For this review, take the finished solid that the model builds, in its own axes (mm). A direction names the side the tool comes from. Give positions to 0.01 mm unless a question says otherwise; leave off trailing zeros. Order: outer loops, then holes, each group sorted by start corner. A loop starts at its lowest first (then second) coordinate and runs counter-clockwise, first axis right, second up. Notation, with made-up numbers: (87.25, 33.25) - (144.25, 33.25) arc R12 ccw to (144.25, 54.25) - close; hole circle Ø5 at (-14.75, 64). An arc over 180 degrees is marked (long way). One line per item, written item: value.
```python
from build123d import *

# Parameters (mm, degrees)
ESBO_O1_R             = 1.25
CORTE_EXTRUS_O1_DEPTH = 10


with BuildPart() as part:
    # Sketch1 → Revolve1 (revolve)
    with BuildSketch(Plane(origin=(0, 0, 0), x_dir=(1, 0, 0), z_dir=(0, 1, 0))):
        Polygon((0, 0), (7, 0), (41.5, 0), (53.5, 0), (53.5, 3), (41.5, 3), (41.5, 3.05), (7, 3.05), (7, 3), (0, 3), align=None)
    revolve(axis=Axis((0, 0, 0), (-1, 0, 0)))

    # Esboço1 → Corte-extrusão1 (cut)
    with BuildSketch(Plane(origin=(53.5, 0, 0), x_dir=(0, 0, -1), z_dir=(1, 0, 0))):
        Circle(ESBO_O1_R)
    extrude(amount=-CORTE_EXTRUS_O1_DEPTH, mode=Mode.SUBTRACT)


solid = part.part
```
(1) For P1, Ø3, axis at x = 44, z = -1.5, coming from the -Y side; P2, Ø1.2, axis at y = -0.5, z = 0, coming from the +X side, all flat-tipped, find the tip position at first contact; note any pin that passes through.
Answers below:
P1: stops at y = -3
P2: stops at x = 43.5
(2) Take a section at A-A (z = 0). Write out the cut boundary in (x, y).
Answers below:
outline: (0, -3) - (7, -3) - (7, -3.05) - (41.5, -3.05) - (41.5, -3) - (53.5, -3) - (53.5, -1.25) - (43.5, -1.25) - (43.5, 1.25) - (53.5, 1.25) - (53.5, 3) - (41.5, 3) - (41.5, 3.05) - (7, 3.05) - (7, 3) - (0, 3) - close
(3) Draft analysis for pull direction Z (two halves, no side actions). For faces 3 (the face through (48.57, -1.22, 0.27)), 4 (the face through (3, 0, 3)), 5 (the face through (0, 0, 0)), state which applies: pulls with the +Z half, pulls with the -Z half, needs draft (parallel to the pull), parting line crosses it, or undercut.
Answers below:
face 3: undercut
face 4: parting line crosses it
face 5: needs draft
(4) Machinability: for faces 1 (the face through (24.008, -0.134, 3.047)), 2 (the face through (47, 0, 3)), which of the approach directions +Z, -Z, +X, -X, +Y, -Y give a long, thin tool a straight path to every point of the face, cutting with its end or side? Answer none if there is none.
Answers below:
face 1: +X, -X
face 2: +X
(5) Take a section at D-D (x = 12.5). Write out the cut boundary in (y, z).
Answers below:
outline: circle Ø6.1 at (0, 0)
(6) Take a section at B-B (x = 44). Write out the cut boundary in (y, z), then the cut area to 3 significant figures.
Answers below:
outline: circle Ø6 at (0, 0); hole circle Ø2.5 at (0, 0)
area: 23.4 mm^2
(7) Wall thickness on line 1 (Y direction, x = 46.25, z = 0); line 2 (Y direction, x = 50.5, z = -1); line 3 (Y direction, x = 10.5, z = 0.5): over which ranges is each line inside the solid? List them lowest first. Write a range as from..to.
Answers below:
line 1: y = -3..-1.25, 1.25..3
line 2: y = -2.83..-0.75, 0.75..2.83
line 3: y = -3.01..3.01
